```python
from build123d import *

# Parameters (mm, degrees)
BOSS_EXTRUDE1_DEPTH = 5
SKETCH2_R           = 2
SKETCH2_W           = 5
SKETCH2_H           = 5
CUT_EXTRUDE1_DEPTH  = 10


with BuildPart() as part:
    # Sketch1 → Boss-Extrude1 (new body)
    with BuildSketch(Plane(origin=(0, 0, 0), x_dir=(1, 0, 0), z_dir=(0, 1, 0))):
        Polygon((44.375484097, 7.788988346), (75.375484097, 7.788988346), (80.375484097, 7.788988346), (80.375484097, 12.788988346), (75.375484097, 12.788988346), (75.375484097, 18.288988346), (73.375484097, 18.288988346), (73.375484097, 17.188988346), (71.075484097, 17.188988346), (71.075484097, 18.288988346), (68.375484097, 18.288988346), (68.375484097, 21.288988346), (71.075484097, 21.288988346), (71.075484097, 22.388988346), (73.375484097, 22.388988346), (73.375484097, 21.288988346), (75.375484097, 21.288988346), (75.375484097, 26.788988346), (80.375484097, 26.788988346), (80.375484097, 31.788988346), (75.375484097, 31.788988346), (44.375484097, 31.788988346), (39.375484097, 31.788988346), (39.375484097, 26.788988346), (44.375484097, 26.788988346), (44.375484097, 21.288988346), (46.375484097, 21.288988346), (46.375484097, 22.388988346), (48.675484097, 22.388988346), (48.675484097, 21.288988346), (51.375484097, 21.288988346), (51.375484097, 18.288988346), (48.675484097, 18.288988346), (48.675484097, 17.188988346), (46.375484097, 17.188988346), (46.375484097, 18.288988346), (44.375484097, 18.288988346), (44.375484097, 12.788988346), (39.375484097, 12.788988346), (39.375484097, 7.788988346), align=None)
    extrude(amount=BOSS_EXTRUDE1_DEPTH)

    # Sketch2 → Cut-Extrude1 (cut)
    with BuildSketch(Plane(origin=(0, 5, 0), x_dir=(1, 0, 0), z_dir=(0, 1, 0))):
        with Locations(Location((59.875484097, 19.788988346, 0), (0, 0, 270))):
            Circle(SKETCH2_R)
        with Locations((59.875484097, 12.288988346)):
            Rectangle(SKETCH2_W, SKETCH2_H)
        with Locations((59.875484097, 27.288988346)):
            Rectangle(SKETCH2_W, SKETCH2_H)
    extrude(amount=-CUT_EXTRUDE1_DEPTH, mode=Mode.SUBTRACT)


solid = part.part
```
The listing builds one solid part. Answer for the finished solid, in the listing's coordinates (mm). A direction names the side the tool comes from. Coordinates: 2 decimals unless noted, no trailing zeros. Loops run counter-clockwise (first coordinate to the right, second up) from the corner with the lowest first, then second, coordinate; pieces in that order, holes last. Notation, with made-up numbers: M 68.25,62.25 L 94.25,62.25 A28 ccw 94.25,80.25 Z; hole C 20,25 d4. An arc over 180 degrees is marked long. Answer as CSV lines item,"result". Start each with the question number.
(1) The part is cut by section A-A (z = -11.25). Give the vertices of the cut face in (x, y), and give its area (3 significant figures).
(2) The mould has two halves that part along Z. Classify faces 4 (the flat face through (60, 2, -31.789)), 5 (the flat face through (60, 3, -9.789)), 6 (the flat face through (60, 5, -23)): pulls with the +Z half, pulls with the -Z half, needs draft (parallel to the pull), parting line crosses it, or undercut.
(3) Given pin 1 (3 mm diameter, centred on x = 59.88, z = -19.79, fed in from +Y); pin 2 (1 mm diameter, centred on y = 3, z = -21, fed in from +X), each flat-ended and moving along its own axis, determine where each tip first touches the part or whether it passes through.
(4) For faces 1 (the flat face through (44.375, 2, -16)), 2 (the flat face through (68.375, 2, -20)), 3 (the flat face through (73.375, 2, -22)), determine the directions among +Z, -Z, +X, -X, +Y, -Y from which every point of the face is accessible in a straight line to the end or side of a thin tool.
(5) Find the intervals of material crossed by L1, parallel to X at y = 0.6, z = -22; L2, parallel to X at y = 0.6, z = -11; L3, parallel to Z at x = 60, y = 1.15, in increasing order. Write a range as [from, to].
(6) The part is cut by section B-B (x = 42). Give the vertices of the cut face in (y, z), and give its area (3 significant figures).
(7) The part is cut by section C-C (x = 58.5). Give the vertices of the cut face in (y, z), and give its area (3 significant figures).
(8) The part is cut by section D-D (y = 1.6). State how many separate pieces and enclosed holes the cut face has, and give its area (3 significant figures).
Determined:
1,outline,"M 39.38,0 L 57.38,0 L 57.38,5 L 39.38,5 Z; M 62.38,0 L 80.38,0 L 80.38,5 L 62.38,5 Z"
1,area,"180 mm2"
2,face 4,"pulls with the -Z half"
2,face 5,"undercut"
2,face 6,"needs draft"
3,pin 1,"through"
3,pin 2,"x = 75.38"
4,face 1,"-X, +Y, -Y"
4,face 2,"+X, +Y, -Y"
4,face 3,"+Y, -Y"
5,L1,"[44.38, 46.38], [48.68, 71.08], [73.38, 75.38]"
5,L2,"[39.38, 57.38], [62.38, 80.38]"
5,L3,"[-31.79, -29.79], [-24.79, -21.79], [-17.79, -14.79], [-9.79, -7.79]"
6,outline,"M 0,-31.79 L 5,-31.79 L 5,-26.79 L 0,-26.79 Z; M 0,-12.79 L 5,-12.79 L 5,-7.79 L 0,-7.79 Z"
6,area,"50.0 mm2"
7,outline,"M 0,-31.79 L 5,-31.79 L 5,-29.79 L 0,-29.79 Z; M 0,-24.79 L 5,-24.79 L 5,-21.24 L 0,-21.24 Z; M 0,-18.34 L 5,-18.34 L 5,-14.79 L 0,-14.79 Z; M 0,-9.79 L 5,-9.79 L 5,-7.79 L 0,-7.79 Z"
7,area,"55.5 mm2"
8,separate pieces,"1"
8,enclosed holes,"3"
8,area,"729 mm2"
